```python
from build123d import *

# Parameters (mm, degrees)
BOSS_EXTRUDE1_DEPTH  = 10
FILLET1_R            = 0.7
FILLET2_R            = 1
FILLET1_OF_MIRROR1_R = 0.7
FILLET2_OF_MIRROR1_R = 1
FILLET3_R            = 4.8


with BuildPart() as part:
    # Sketch1 → Boss-Extrude1 (new body)
    with BuildSketch(Plane(origin=(0, 0, 0), x_dir=(1, 0, 0), z_dir=(0, 1, 0))):
        Polygon((0, 0), (-5, 0), (-11, -7.2), (-3.75, -7.2), (-3.75, -12.2), (0, -12.2), align=None)
    boss_extrude1 = extrude(amount=BOSS_EXTRUDE1_DEPTH)

    # Fillet1
    fillet1_edges = [part.edges().sort_by_distance(p)[0] for p in [
        (-11, 5, 7.2),
    ]]
    fillet(fillet1_edges, radius=FILLET1_R)

    # Fillet2
    fillet2_edges = [part.edges().sort_by_distance(p)[0] for p in [
        (-3.75, 5, 7.2),
    ]]
    fillet(fillet2_edges, radius=FILLET2_R)

    # Mirror1: Boss-Extrude1 across plane
    add(boss_extrude1.mirror(Plane(origin=(0, 10, 12.2), x_dir=(0, 0, 1), z_dir=(-1, 0, 0))))

    # Fillet1 of Mirror1
    fillet1_of_mirror1_edges = [part.edges().sort_by_distance(p)[0] for p in [
        (11, 5, 7.2),
    ]]
    fillet(fillet1_of_mirror1_edges, radius=FILLET1_OF_MIRROR1_R)

    # Fillet2 of Mirror1
    fillet2_of_mirror1_edges = [part.edges().sort_by_distance(p)[0] for p in [
        (3.75, 5, 7.2),
    ]]
    fillet(fillet2_of_mirror1_edges, radius=FILLET2_OF_MIRROR1_R)

    # Fillet3
    fillet3_edges = [part.edges().sort_by_distance(p)[0] for p in [
        (-5, 5, 0),
        (5, 5, 0),
    ]]
    fillet(fillet3_edges, radius=FILLET3_R)


solid = part.part
```
Source: CAD feature listing. Evaluate the final solid. Frame: model axes, mm. A direction names the side the tool comes from. Round coordinates to 2 decimals unless told otherwise and drop trailing zeros. Order: outer loops, then holes, each group sorted by start corner. A loop starts at its lowest first (then second) coordinate and runs counter-clockwise, first axis right, second up. Notation, with made-up numbers: (30.25, 44.25) -> (83.25, 44.25) arc R24 cw to (83.25, 81.25) -> close; hole circle Ø2 at (33.5, -16). An arc over 180 degrees is marked (long way). One line per item, written item: value. Start each with the question number.
Q1. Section query C-C (z = 9.75). Return the cut outline in (x, y).
Q2. Pin query (flat end, axial travel): pin 1 (3 mm diameter, centred on y = 3.5, z = 9.5, fed in from +X); pin 2 (5 mm diameter, centred on y = 7.5, z = 10, fed in from +X); pin 3 (3 mm diameter, centred on y = 6.5, z = 10, fed in from -X). Return the tip coordinate at first contact, or that it passes through.
Q3. Material intervals for probe 1 along X at (y, z) = (5.75, 9.25); probe 2 along X at (y, z) = (7.25, 2.5); probe 3 along Z at (x, y) = (-5.5, 9.25), sorted ascending.
Q4. Access query for faces 1 (the flat face through (-3.75, 5, 10)), 2 (the flat face through (7, 5, 7.2)), 3 (the flat face through (8.216, 4.93, 3.859)). Directions: +Z, -Z, +X, -X, +Y, -Y. A direction counts if a zero-diameter tool reaches every point of the face in a straight line with its end or side. Return the directions, or none.
Q5. Section query A-A (y = 5.75). Return the cut outline in (x, z), plus the area to 3 significant figures.
Q6. Section query B-B (x = 7.5). Return the cut outline in (y, z).
Findings below:
1. outline: (-3.75, 0) -> (3.75, 0) -> (3.75, 10) -> (-3.75, 10) -> close
2. pin 1: x = 3.77
2. pin 2: x = 4.04
2. pin 3: x = -3.75
3. probe 1: -3.75 to 3.75
3. probe 2: -7.08 to 7.08
3. probe 3: 0.86 to 7.2
4. face 1: +Z, -X, +Y, -Y
4. face 2: +Z, +X, +Y, -Y
4. face 3: -Z, +X, +Y, -Y
5. outline: (-10.04, 6.05) -> (-6.44, 1.73) arc R4.8 ccw to (-2.75, 0) -> (2.75, 0) arc R4.8 ccw to (6.44, 1.73) -> (10.04, 6.05) arc R0.7 ccw to (9.51, 7.2) -> (4.75, 7.2) arc R1 cw to (3.75, 8.2) -> (3.75, 12.2) -> (-3.75, 12.2) -> (-3.75, 8.2) arc R1 cw to (-4.75, 7.2) -> (-9.51, 7.2) arc R0.7 ccw to start
5. area: 151 mm²
6. outline: (0, 3) -> (10, 3) -> (10, 7.2) -> (0, 7.2) -> close
